Geometry: final body of the model. Coordinates: model frame, mm. A direction names the side the tool comes from. Give positions to 0.01 mm unless a question says otherwise; leave off trailing zeros. Loops run counter-clockwise (first coordinate to the right, second up) from the corner with the lowest first, then second, coordinate; pieces in that order, holes last. Notation, with made-up numbers: M 58,61.25 L 84,61.25 A26 ccw 84,84.25 Z; hole C -4,69 d7. An arc over 180 degrees is marked long. Put each result on its own line as item: value.
Autodesk Inventor part; units mm, degrees
ref_plane "YZ Plane" through (0, 0, 0) normal (1, 0, 0) x (0, 1, 0)
ref_plane "XZ Plane" through (0, 0, 0) normal (0, 1, 0) x (-1, 0, 0)
ref_plane "XY Plane" through (0, 0, 0) normal (0, 0, 1) x (1, 0, 0)
sketch "Skizze1" plane through (0, 0, 0) normal (0, 0, 1) x (1, 0, 0)
  line L0 (140.5121, 9.5998) -> (90.5121, 9.5998)
  line L1 (90.5121, 9.5998) -> (90.5121, 21.5998)
  line L2 (90.5121, 21.5998) -> (140.5121, 21.5998)
  line L3 (140.5121, 21.5998) -> (140.5121, 9.5998)
  point P0 (0, 0)
  dimension "d0" = 50
  dimension "d1" = 12
extrude "Extrusion1" add sketch "Skizze1" along normal blind 30
sketch "Skizze2" plane through (0, 0, 30) normal (0, 0, 1) x (1, 0, 0)
  line L0 (140.5121, 9.5998) -> (140.5121, 21.5998)
  line L1 (140.5121, 14.5998) -> (133.5121, 14.5998)
  line L2 (133.5121, 14.5998) -> (97.5121, 14.5998)
  line L3 (97.5121, 14.5998) -> (90.5121, 14.5998)
  line L4 (90.5121, 21.5998) -> (90.5121, 9.5998)
  line L5 (140.5121, 21.5998) -> (90.5121, 21.5998)
  point P0 (0, 0)
  dimension "d4" = 7
  dimension "d12" = 7
hole "Bohrung1" at (133.5121, 14.5998, 30) at (97.5121, 14.5998, 30) direction (0, 0, -1) diameter 4.3 end through all countersink diameter 9.4 countersink angle 90
sketch "Skizze3" plane through (90.5121, 9.5998, 0) normal (0, 1, 0) x (1, 0, 0)
  line L0 (25, -23) -> (25, -30)
  line L1 (50, -30) -> (0, -30)
  point P0 (-90.5121, 0)
  dimension "d14" = 7
hole "Bohrung4" at (115.5121, 9.5998, 23) direction (0, 1, 0) diameter 3.242 depth 10 tip angle 118
fillet "Rundung2" radius 2 5 edges at (140.5121, 15.5998, 30) (115.5121, 21.5998, 30) (90.5121, 15.5998, 30) (140.5121, 21.5998, 15) (90.5121, 21.5998, 15)
properties part number "HebelhalterBlock" material "Aluminium 6061(1)"
Item 1: Pin query (flat end, axial travel): pin 1 Ø5.5 at (x, y) = (97.51, 14.6) entering from +Z; pin 2 Ø4 at (x, y) = (133.51, 14.6) entering from +Z. Return the tip coordinate at first contact, or that it passes through.
Output values:
pin 1: z = 28.05
pin 2: through
Item 2: Section A-A on z = 3.25. Output: boundary loops of the cut face in (x, y).
Output values:
outline: M 90.51,9.6 L 140.51,9.6 L 140.51,19.6 A2 ccw 138.51,21.6 L 92.51,21.6 A2 ccw 90.51,19.6 Z; hole C 97.51,14.6 d4.3; hole C 133.51,14.6 d4.3
Item 3: Section B-B on y = 16.25. Count the separate pieces of the cut face and the enclosed holes in it, then the cut area to 3 significant figures.
Output values:
separate pieces: 3
enclosed holes: 1
area: 1,310 mm²
Item 4: Line query: probe 1 along X at (y, z) = (14.5, 3); probe 2 along X at (y, z) = (14.25, 7.5); probe 3 along X at (y, z) = (13.5, 23). Output: solid intervals per line, ascending. Write a range as [from, to].
Output values:
probe 1: [90.51, 95.36], [99.66, 131.36], [135.66, 140.51]
probe 2: [90.51, 95.39], [99.63, 131.39], [135.63, 140.51]
probe 3: [90.51, 95.66], [99.36, 113.89], [117.13, 131.66], [135.36, 140.51]
Item 5: Mould query, pull axis Y, two halves, no side actions, for faces 3 (the conical face through (115.237, 20.405, 23.061)), 4 (the cylindrical face through (139.94, 14.53, 29.4)), 5 (the cylindrical face through (115.83, 21.03, 29.4)), 6 (the cylindrical face through (135.61, 15.07, 13.53)). Classes: pulls with the +Y half, pulls with the -Y half, needs draft (parallel to the pull), parting line crosses it, or undercut.
Output values:
face 3: pulls with the -Y half
face 4: needs draft
face 5: pulls with the +Y half
face 6: undercut
Item 6: Set-up query: faces 1 (the cylindrical face through (113.905, 14.67, 23.211)), 2 (the flat face through (116, 9.6, 15)). Return all of +Z, -Z, +X, -X, +Y, -Y with unobstructed straight access to the full face (end or side cutting, diameter ignored); none if empty.
Output values:
face 1: -Y
face 2: +Z, -Z, +X, -X, -Y
